For this review, take the finished solid that the model builds, in its own axes (mm). Round coordinates to 2 decimals unless told otherwise and drop trailing zeros. Order: outer loops, then holes, each group sorted by start corner. A loop starts at its lowest first (then second) coordinate and runs counter-clockwise, first axis right, second up. Notation, with made-up numbers: (-26, 71.5) -> (0, 71.5) arc R23 cw to (0, 83.5) -> close; hole circle Ø2 at (70, -0.5). An arc over 180 degrees is marked (long way). Answer in a Markdown table with one row per item.
```python
from build123d import *

# Parameters (mm, degrees)
SKETCH_1_W      = 200
SKETCH_1_H      = 280
SKETCH_1_R      = 7.5
SKETCH_1_W_2    = 5
SKETCH_1_H_2    = 90
EXTRUDE_1_DEPTH = 3


with BuildPart() as part:
    # 草圖1 → 填料-伸長1 (new body)
    with BuildSketch(Plane.XY):
        Rectangle(SKETCH_1_W, SKETCH_1_H)
        with Locations((0, 40)):
            Circle(SKETCH_1_R, mode=Mode.SUBTRACT)
        with Locations((-91.5, -2)):
            Rectangle(SKETCH_1_W_2, SKETCH_1_H_2, mode=Mode.SUBTRACT)
    extrude(amount=EXTRUDE_1_DEPTH)


solid = part.part
```
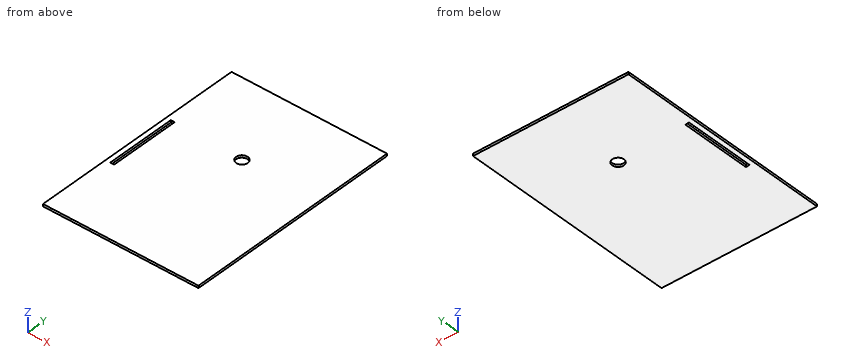
Q1. Take a section at A-A, the plane y = 40. Write out the cut boundary in (x, z), then the cut area to 3 significant figures.
Answer key:
| item | result |
|---|---|
| outline | (-100, 0) -> (-94, 0) -> (-94, 3) -> (-100, 3) -> close; (-89, 0) -> (-7.5, 0) -> (-7.5, 3) -> (-89, 3) -> close; (7.5, 0) -> (100, 0) -> (100, 3) -> (7.5, 3) -> close |
| area | 540 mm^2 |
Q2. Take a section at C-C, the plane y = -1.5. Write out the cut boundary in (x, z), then the cut area to 3 significant figures.
Answer key:
| item | result |
|---|---|
| outline | (-100, 0) -> (-94, 0) -> (-94, 3) -> (-100, 3) -> close; (-89, 0) -> (100, 0) -> (100, 3) -> (-89, 3) -> close |
| area | 585 mm^2 |
Q3. Clearance check with a flat-ended pin moving along its axis: pin 1 Ø13.5 at (x, y) = (0, 40) entering from -Z. State where the tip first meets the part, or that it passes through.
Answer key:
| item | result |
|---|---|
| pin 1 | passes through |
Q4. To check wall thickness, follow probe 1 along Y at (x, z) = (0, 1.7); probe 2 along X at (y, z) = (-33, 2); probe 3 along Y at (x, z) = (3, 1.05). State the ranges of each line that lie inside material, in increasing order.
Answer key:
| item | result |
|---|---|
| probe 1 | y = -140 to 32.5, 47.5 to 140 |
| probe 2 | x = -100 to -94, -89 to 100 |
| probe 3 | y = -140 to 33.13, 46.87 to 140 |
Q5. Take a section at B-B, the plane x = 0. Write out the cut boundary in (y, z), then the cut area to 3 significant figures.
Answer key:
| item | result |
|---|---|
| outline | (-140, 0) -> (32.5, 0) -> (32.5, 3) -> (-140, 3) -> close; (47.5, 0) -> (140, 0) -> (140, 3) -> (47.5, 3) -> close |
| area | 795 mm^2 |
